Part print with two shaded views. Sizes in mm from the minimum x, y, z corner. A direction names the side the tool comes from. Round coordinates to 2 decimals unless told otherwise and drop trailing zeros. Write each loop counter-clockwise with the first axis right and the second up, starting at its lowest first coordinate (ties: lowest second). Pieces come first, ordered by that corner, then holes. Notation, with made-up numbers: (-0.75, 60) -> (42.25, 60) arc R32 ccw to (42.25, 96) -> close; hole circle Ø10 at (37.5, -36). An arc over 180 degrees is marked (long way). Return JSON: item names as keys, results as strings.
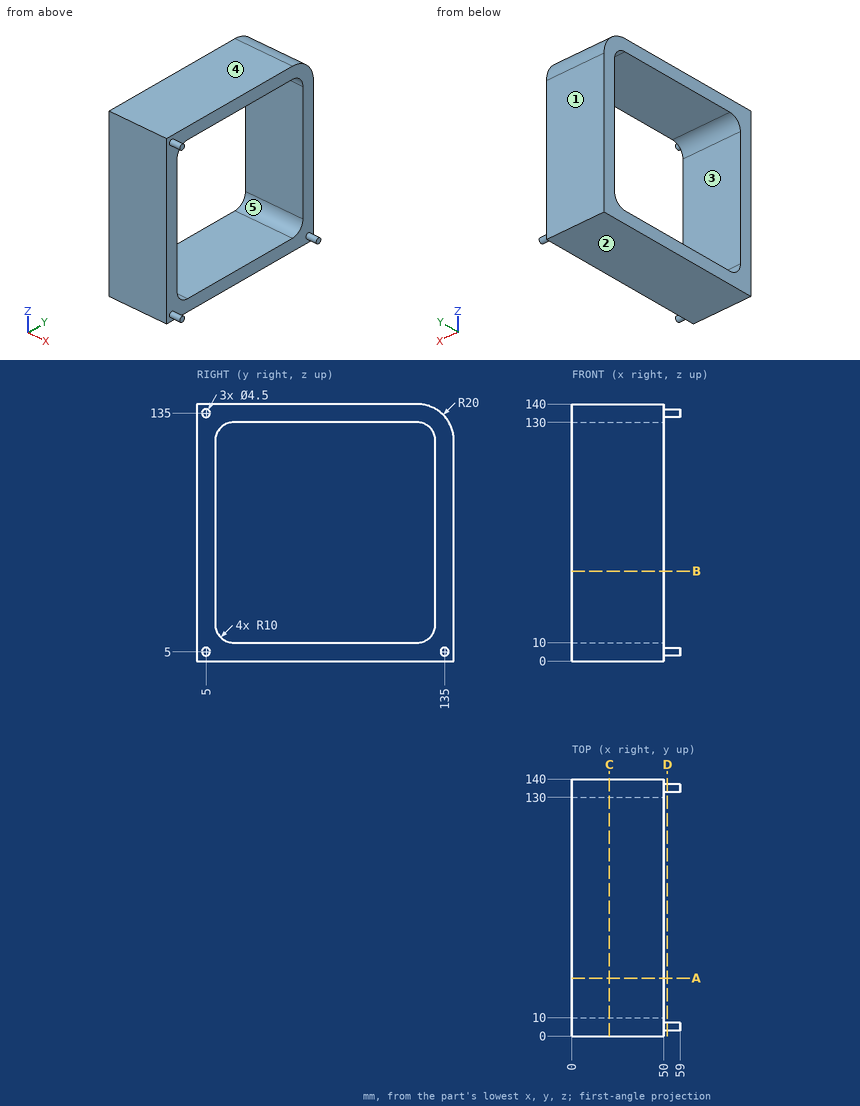
Q1. Saw through at D-D on x = 52. List the corners of the cut face in (y, z), then the cut area to 3 significant figures.
Verdict:
{"outline": "circle Ø4.5 at (5, 5); circle Ø4.5 at (5, 135); circle Ø4.5 at (135, 5)", "area": "47.7 mm²"}
Q2. Wall check: L1, parallel to Y at x = 21.5, z = 103; L2, parallel to X at y = 131, z = 102.5. Give the ranges that are in metal, low to high.
Verdict:
{"L1": "y = 0 to 10, 130 to 140", "L2": "x = 0 to 50"}
Q3. Saw through at A-A on y = 31.5. List the corners of the cut face in (x, z), then the cut area to 3 significant figures.
Verdict:
{"outline": "(0, 0) -> (50, 0) -> (50, 10) -> (0, 10) -> close; (0, 130) -> (50, 130) -> (50, 140) -> (0, 140) -> close", "area": "1,000 mm²"}
Q4. 3-axis set-ups, long thin cutter, end or side, ignore diameter. For the marked faces 4 and 5: which of +Z, -Z, +X, -X, +Y, -Y reach the whole face in a straight line?
Verdict:
{"face 4": "+Z, +X, -X, +Y, -Y", "face 5": "+X, -X"}
Q5. Saw through at C-C on x = 20.5. List the corners of the cut face in (y, z).
Verdict:
{"outline": "(0, 0) -> (140, 0) -> (140, 120) arc R20 ccw to (120, 140) -> (0, 140) -> close; hole (10, 20) arc R10 ccw to (20, 10) -> (120, 10) arc R10 ccw to (130, 20) -> (130, 120) arc R10 ccw to (120, 130) -> (20, 130) arc R10 ccw to (10, 120) -> close"}
Q6. Pin check, flat tip, straight feed: pin 1 Ø1.5 at (x, z) = (21.5, 66) entering from -Y. Stop position of the tip, or through.
Verdict:
{"pin 1": "stops at y = 0"}
Q7. Two-plate mould, pull along Y, no slides. Class the marked faces 1, 2 and 3: +Y half, -Y half, draft (parallel to the pull), parting line (faces both ways), or undercut.
Verdict:
{"face 1": "+Y half", "face 2": "draft", "face 3": "undercut"}
